Geometry check sheet. Reference: the model listing, model coordinates, mm. A direction names the side the tool comes from. Round coordinates to 2 decimals unless told otherwise and drop trailing zeros. Write each loop counter-clockwise with the first axis right and the second up, starting at its lowest first coordinate (ties: lowest second). Pieces come first, ordered by that corner, then holes.
Item 1: Draft check along X on faces 1 (the face through (13, 0, 3)), 2 (the face through (32.5, 0, 5)), 3 (the face through (0, -13, 3)), 4 (the face through (0, 32.5, 5)). Enter one of: pulls with the +X half, pulls with the -X half, needs draft (parallel to the pull), parting line crosses it, or undercut.
Item 2: Cross-section at C-C (z = 18). Enter the section's corners in (x, y), then the cut area to 3 significant figures.
Item 3: Access from +Z, -Z, +X, -X, +Y, -Y to the whole of each face (thin tool, end or side, straight path). Record for faces 5 (the face through (-25, 0, 12)), 6 (the face through (0, -12.5, 17)), 7 (the face through (12.5, 0, 17)).
Item 4: Cross-section at D-D (x = 31). Enter the section's corners in (y, z), then the cut area to 3 significant figures.
Item 5: Depth check by flat-ended pin: P1, Ø5.5, axis at x = -3, z = 17, coming from the +Y side; P2, Ø2, axis at x = 2, z = 6.5, coming from the +Y side; P3, Ø6, axis at y = -5.5, z = 15.5, coming from the +X side. Enter the tip coordinate at first touch or a pass-through.
Item 6: Scan lines: probe 1 along X at (y, z) = (3.5, 3.5); probe 2 along X at (y, z) = (21.5, 3.5); probe 3 along X at (y, z) = (0, 12.25). Record each from-to range of solid material in increasing order.
Solid Edge part; units mm, degrees
sketch "Sketch1" plane through (0, 0, 0) normal (0, 0, 1) x (1, 0, 0)
  line L0 (-37.5, -37.5) -> (37.5, -37.5)
  line L1 (37.5, -37.5) -> (37.5, 37.5)
  line L2 (37.5, 37.5) -> (-37.5, 37.5)
  line L3 (-37.5, 37.5) -> (-37.5, -37.5)
extrude "Protrusion1" add sketch "Sketch1" along normal blind 2
sketch "Sketch2" plane through (0, 0, 0) normal (0, 0, 1) x (1, 0, 0)
  line L0 (-35, -35) -> (35, -35)
  line L1 (35, -35) -> (35, 35)
  line L2 (35, 35) -> (-35, 35)
  line L3 (-35, 35) -> (-35, -35)
extrude "ExtrudedProtrusion_2" add sketch "Sketch2" along normal blind 4
sketch "Sketch3" plane through (0, 0, 0) normal (0, 0, 1) x (1, 0, 0)
  line L0 (-32.5, -32.5) -> (32.5, -32.5)
  line L1 (32.5, -32.5) -> (32.5, 32.5)
  line L2 (32.5, 32.5) -> (-32.5, 32.5)
  line L3 (-32.5, 32.5) -> (-32.5, -32.5)
extrude "ExtrudedProtrusion_3" add sketch "Sketch3" along normal blind 6
sketch "Sketch4" plane through (0, 0, 0) normal (0, 0, 1) x (1, 0, 0)
  line L0 (-30, -30) -> (30, -30)
  line L1 (30, -30) -> (30, 30)
  line L2 (30, 30) -> (-30, 30)
  line L3 (-30, 30) -> (-30, -30)
extrude "ExtrudedProtrusion_4" add sketch "Sketch4" along normal blind 8
sketch "Sketch5" plane through (0, 0, 0) normal (0, 0, 1) x (1, 0, 0)
  line L0 (-27.5, -27.5) -> (27.5, -27.5)
  line L1 (27.5, -27.5) -> (27.5, 27.5)
  line L2 (27.5, 27.5) -> (-27.5, 27.5)
  line L3 (-27.5, 27.5) -> (-27.5, -27.5)
extrude "ExtrudedProtrusion_5" add sketch "Sketch5" along normal blind 10
sketch "Sketch6" plane through (0, 0, 0) normal (0, 0, 1) x (1, 0, 0)
  line L0 (-25, 25) -> (-25, -25)
  line L1 (-25, -25) -> (25, -25)
  line L2 (25, -25) -> (25, 25)
  line L3 (25, 25) -> (-25, 25)
extrude "ExtrudedProtrusion_6" add sketch "Sketch6" along normal blind 15
sketch "Sketch7" plane through (0, 0, 0) normal (0, 0, 1) x (1, 0, 0)
  line L0 (13, 13) -> (-13, 13)
  line L1 (-13, 13) -> (-13, -13)
  line L2 (-13, -13) -> (13, -13)
  line L3 (13, -13) -> (13, 13)
extrude "ExtrudedCutout_1" cut sketch "Sketch7" along normal blind 5.5
sketch "Sketch8" plane through (0, 0, 15) normal (0, 0, 1) x (0, -1, 0)
  line L0 (-12.5, -12.5) -> (12.5, -12.5)
  line L1 (12.5, -12.5) -> (12.5, 12.5)
  line L2 (12.5, 12.5) -> (-12.5, 12.5)
  line L3 (-12.5, 12.5) -> (-12.5, -12.5)
extrude "ExtrudedProtrusion_8" add sketch "Sketch8" along normal blind 5
Resolved:
1. face 1: undercut
1. face 2: pulls with the +X half
1. face 3: undercut
1. face 4: needs draft
2. outline: (-12.5, -12.5) - (12.5, -12.5) - (12.5, 12.5) - (-12.5, 12.5) - close
2. area: 625 mm2
3. face 5: +Z, -X, +Y, -Y
3. face 6: +Z, +X, -X, -Y
3. face 7: +Z, +X, +Y, -Y
4. outline: (-37.5, 0) - (37.5, 0) - (37.5, 2) - (35, 2) - (35, 4) - (32.5, 4) - (32.5, 6) - (-32.5, 6) - (-32.5, 4) - (-35, 4) - (-35, 2) - (-37.5, 2) - close
4. area: 420 mm2
5. P1: stops at y = 25
5. P2: stops at y = 32.5
5. P3: stops at x = 25
6. probe 1: x = -35 to -13, 13 to 35
6. probe 2: x = -35 to 35
6. probe 3: x = -25 to 25
